Here's how the part is built. I have some questions about the finished solid (model axes, mm). Coordinates: 2 decimals unless noted, no trailing zeros. Loops run counter-clockwise (first coordinate to the right, second up) from the corner with the lowest first, then second, coordinate; pieces in that order, holes last. Notation, with made-up numbers: M 78,11 L 137,11 A28 ccw 137,47 Z; hole C 29,-24 d9. An arc over 180 degrees is marked long. Use CSV: the item, a comma, the result in double quotes. Start each with the question number.
Q1. If we section it at B-B (y = 5): Please give me the cut outline in (x, z).
Q2. If we mould it in two halves opening along X, with no side actions, what happens to faces 1 (the flat face through (35, 5, 2)), 2 (the flat face through (13, 14, 0)), 3 (the cylindrical face through (5, 28, 3)), 4 (the cylindrical face through (31.908, 5.601, 2.535))? For each: +X half, -X half, draft (parallel to the pull), parting line (faces both ways), or undercut.
Q3. If we section it at A-A (x = 30): Please give me the cut outline in (y, z).
Q4. Please list where these lines run through material, in increasing order: probe 1 along Y at (x, z) = (5, 2.7); probe 2 along X at (y, z) = (5.5, 3.8); probe 3 along Y at (x, z) = (30, 2.1). Write a range as [from, to].
Q5. If we section it at C-C (y = 14): Please give me the cut outline in (x, z).
Q6. If we section it at D-D (z = 2.1): Please give me the cut outline in (x, y).
from build123d import *

# Parameters (mm, degrees)
BOSS_EXTRU_1_DEPTH      = 5
ESQUISSE2_R             = 2
ENL_V_MAT_EXTRU_1_DEPTH = 5


with BuildPart() as part:
    # Esquisse1 → Boss.-Extru.1 (new body)
    with BuildSketch(Plane.XY):
        Polygon((0, 0), (35, 0), (35, 10), (10, 35), (0, 35), align=None)
    extrude(amount=BOSS_EXTRU_1_DEPTH)

    # Esquisse2 → Enlèv. mat.-Extru.1 (cut)
    with BuildSketch(Plane.XY.offset(5)):
        with Locations((14, 5)):
            Circle(ESQUISSE2_R)
        with Locations((30, 5)):
            Circle(ESQUISSE2_R)
        with Locations((5, 30)):
            Circle(ESQUISSE2_R)
        with Locations((5, 14)):
            Circle(ESQUISSE2_R)
    extrude(amount=-ENL_V_MAT_EXTRU_1_DEPTH, mode=Mode.SUBTRACT)


solid = part.part
Results below:
1,outline,"M 0,0 L 12,0 L 12,5 L 0,5 Z; M 16,0 L 28,0 L 28,5 L 16,5 Z; M 32,0 L 35,0 L 35,5 L 32,5 Z"
2,face 1,"+X half"
2,face 2,"draft"
2,face 3,"undercut"
2,face 4,"undercut"
3,outline,"M 0,0 L 3,0 L 3,5 L 0,5 Z; M 7,0 L 15,0 L 15,5 L 7,5 Z"
4,probe 1,"[0, 12], [16, 28], [32, 35]"
4,probe 2,"[0, 12.06], [15.94, 28.06], [31.94, 35]"
4,probe 3,"[0, 3], [7, 15]"
5,outline,"M 0,0 L 3,0 L 3,5 L 0,5 Z; M 7,0 L 31,0 L 31,5 L 7,5 Z"
6,outline,"M 0,0 L 35,0 L 35,10 L 10,35 L 0,35 Z; hole C 5,14 d4; hole C 5,30 d4; hole C 14,5 d4; hole C 30,5 d4"
